```python
from build123d import *

# Parameters (mm, degrees)
F1_DEPTH = 5
F0_W     = 13
F0_H     = 13
F0_R     = 4
F0_R_2   = 2.25
F2_DEPTH = 10
F3_DEPTH = 13
F4_DEPTH = 6
F5_SIZE  = 2
F6_R     = 3
F7_R     = 2
F8_R     = 5
F11_R    = 15


with BuildPart() as f1:
    # F0 (on Top) → F1 (new body)
    with BuildSketch(Plane.XY):
        with BuildLine():
            ThreePointArc((43.1918518623, 30.1804338837), (45.0913645201, 31.5395055678), (46.65, 29.8))
            ThreePointArc((46.65, 29.8), (46.3207025236, 28.7781857608), (45.4567378977, 28.1409210648))
            Line((45.4567378977, 28.1409210648), (47.2860195617, 22.6896617063))
            Line((47.2860195617, 22.6896617063), (54.9, 0))
            Line((54.9, 0), (64.9, 0))
            Line((64.9, 0), (64.9, 33.8))
            Line((64.9, 33.8), (61.9, 33.8))
            Line((61.9, 33.8), (48.9, 33.8))
            Line((48.9, 33.8), (48.9, 46.8))
            Line((48.9, 46.8), (48.9, 49.8))
            Line((48.9, 49.8), (0, 49.8))
            Line((0, 49.8), (0, 39.8))
            Line((0, 39.8), (37.5793651244, 31.43043093))
            Line((37.5793651244, 31.43043093), (43.1918518623, 30.1804338837))
        make_face()
        with BuildLine():
            ThreePointArc((45.4567378977, 28.1409210648), (43.7289579343, 28.499553738), (43.1918518623, 30.1804338837))
            Line((43.1918518623, 30.1804338837), (37.5793651244, 31.43043093))
            ThreePointArc((37.5793651244, 31.43043093), (39.8812482897, 24.2266588773), (47.2860195617, 22.6896617063))
            Line((47.2860195617, 22.6896617063), (45.4567378977, 28.1409210648))
        make_face()
    extrude(amount=F1_DEPTH)

    # F0 (on Top) → F2 (join)
    with BuildSketch(Plane.XY):
        with Locations((55.4, 40.3)):
            Rectangle(F0_W, F0_H)
        with Locations((55.8, 40.6)):
            Circle(F0_R, mode=Mode.SUBTRACT)
        with Locations((55.8, 40.6)):
            Circle(F0_R)
        with Locations((55.8, 40.6)):
            Circle(F0_R_2, mode=Mode.SUBTRACT)
    extrude(amount=F2_DEPTH)

    # F0 (on Top) → F3 (join)
    with BuildSketch(Plane.XY):
        Polygon((64.9, 49.8), (48.9, 49.8), (48.9, 46.8), (61.9, 46.8), (61.9, 33.8), (64.9, 33.8), align=None)
    extrude(amount=F3_DEPTH)

    # F0 (on Top) → F4 (cut)
    with BuildSketch(Plane.XY):
        with Locations((55.8, 40.6)):
            Circle(F0_R)
        with Locations((55.8, 40.6)):
            Circle(F0_R_2, mode=Mode.SUBTRACT)
    extrude(amount=F4_DEPTH, mode=Mode.SUBTRACT)

    # F5
    f5_edges = [f1.edges().sort_by_distance(p)[0] for p in [
        (43.15, 29.8, 5),
    ]]
    chamfer(f5_edges, length=F5_SIZE)

    # F6
    f6_edges = [f1.edges().sort_by_distance(p)[0] for p in [
        (48.9, 33.8, 7.5),
    ]]
    fillet(f6_edges, radius=F6_R)

    # F7
    f7_edges = [f1.edges().sort_by_distance(p)[0] for p in [
        (58.4, 33.8, 5),
        (49.77868, 34.67868, 5),
        (48.9, 43.3, 5),
    ]]
    fillet(f7_edges, radius=F7_R)

    # F8
    f8_edges = [f1.edges().sort_by_distance(p)[0] for p in [
        (37.579365, 31.430431, 2.5),
        (47.28602, 22.689662, 2.5),
    ]]
    fillet(f8_edges, radius=F8_R)

    # F9: F1 across face


with BuildPart() as f1_1:
    add(f1.part)
    add(f1.part.mirror(Plane(origin=(0, 44.8, 2.5), x_dir=(0, -1, 0), z_dir=(-1, 0, 0))))

    # F10: F1 across face


with BuildPart() as f1_2:
    add(f1_1.part)
    add(f1_1.part.mirror(Plane(origin=(59.9, 0, 2.5), x_dir=(1, 0, 0), z_dir=(0, -1, 0))))

    # F11
    f11_edges = [f1_2.edges().sort_by_distance(p)[0] for p in [
        (0, 39.8, 2.5),
        (54.9, 0, 2.5),
        (0, -39.8, 2.5),
        (-54.9, 0, 2.5),
    ]]
    fillet(f11_edges, radius=F11_R)


solid = f1_2.part
```
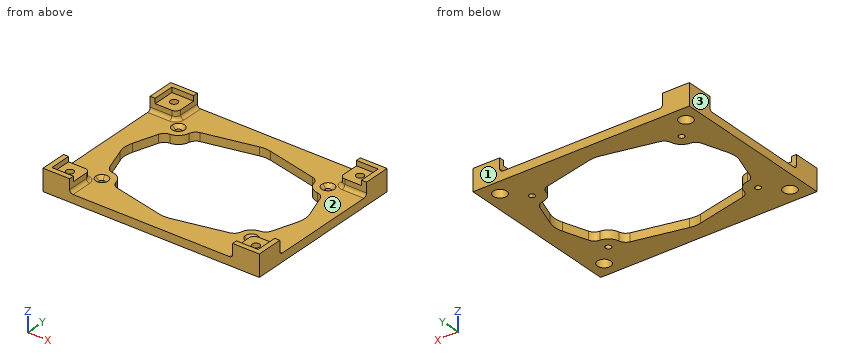
Input: part model. Units: mm. Frame: model coordinates. Face numbers are marked on the shaded views. Give positions to 0.01 mm unless a question says otherwise; leave off trailing zeros. Order: outer loops, then holes, each group sorted by start corner. A loop starts at its lowest first (then second) coordinate and runs counter-clockwise, first axis right, second up.
1. Pin query (flat end, axial travel): pin 1 (2.5 mm diameter, centred on x = 55.5, y = -42.5, fed in from -Z); pin 2 (4 mm diameter, centred on x = 58.5, y = -42, fed in from +Z). Return the tip coordinate at first contact, or that it passes through.
Derived:
pin 1: stops at z = 6
pin 2: stops at z = 10
2. Mould query, pull axis X, two halves, no side actions, for the marked faces 1, 2 and 3. Classes: released by +X, released by -X, zero draft, split by the parting line, or undercut.
Derived:
face 1: zero draft
face 2: undercut
face 3: released by -X
3. Section C-C on y = -16.5. Return the cut outline in (x, z).
Derived:
outline: (-64.9, 0) - (-49.36, 0) - (-49.36, 5) - (-64.9, 5) - close; (49.36, 0) - (64.9, 0) - (64.9, 5) - (49.36, 5) - close
4. Section A-A on x = 55.8. Give the number of separate pieces and of enclosed holes in the cut face, and give its area (3 significant figures).
Derived:
separate pieces: 3
enclosed holes: 0
area: 546 mm2
5. Section D-D on x = 19.5. Return the cut outline in (y, z), and give its area (3 significant figures).
Derived:
outline: (-49.8, 0) - (-35.46, 0) - (-35.46, 5) - (-49.8, 5) - close; (35.46, 0) - (49.8, 0) - (49.8, 5) - (35.46, 5) - close
area: 143 mm2
6. Section B-B on z = 11.5. Return the cut outline in (x, y), and give its area (3 significant figures).
Derived:
outline: (-64.9, -49.8) - (-48.9, -49.8) - (-48.9, -46.8) - (-61.9, -46.8) - (-61.9, -33.8) - (-64.9, -33.8) - close; (-64.9, 33.8) - (-61.9, 33.8) - (-61.9, 46.8) - (-48.9, 46.8) - (-48.9, 49.8) - (-64.9, 49.8) - close; (48.9, -49.8) - (64.9, -49.8) - (64.9, -33.8) - (61.9, -33.8) - (61.9, -46.8) - (48.9, -46.8) - close; (48.9, 46.8) - (61.9, 46.8) - (61.9, 33.8) - (64.9, 33.8) - (64.9, 49.8) - (48.9, 49.8) - close
area: 348 mm2
7. Material intervals for L1, parallel to X at y = -40.6, z = 1.45; L2, parallel to Y at x = 55.8, z = 2.1; L3, parallel to Y at x = -55.8, z = 7.45, sorted ascending.
Derived:
L1: x = -64.9 to -59.8, -51.8 to 51.8, 59.8 to 64.9
L2: y = -49.8 to -44.6, -36.6 to 36.6, 44.6 to 49.8
L3: y = -49.8 to -42.85, -38.35 to -33.8, 33.8 to 38.35, 42.85 to 49.8
